```python
from build123d import *

# Parameters (mm, degrees)
EXTRUDE_1_DEPTH     = 332
SKETCH_2_R          = 3.25
CUT_EXTRUDE_1_DEPTH = 5
SKETCH_3_R          = 5
CUT_EXTRUDE_2_DEPTH = 5
SKETCH_4_W          = 26.179083289
SKETCH_4_H          = 3.25731829
CUT_EXTRUDE_3_DEPTH = 10
SKETCH_5_R          = 1.75
CUT_EXTRUDE_4_DEPTH = 2.5
CHAMFER_1_SIZE      = 1.5
SKETCH_6_R          = 2.1
SKETCH_6_R_2        = 6
CUT_EXTRUDE_5_DEPTH = 10
SKETCH_8_R          = 2.1
SKETCH_8_R_2        = 1.1
CUT_EXTRUDE_6_DEPTH = 10
SKETCH_9_R          = 1.6
CUT_EXTRUDE_7_DEPTH = 10
CHAMFER_2_SIZE      = 1.5
SKETCH_10_R         = 2.1
CUT_EXTRUDE_8_DEPTH = 10


with BuildPart() as part:
    # Эскиз1 → Вытянуть1 (new body)
    with BuildSketch(Plane.XY):
        with BuildLine():
            Line((-1, -68), (-1, 104))
            ThreePointArc((-1, 104), (0.171572875, 106.828427125), (3, 108))
            Line((3, 108), (24, 108))
            Line((24, 108), (24, 106))
            Line((24, 106), (3, 106))
            ThreePointArc((3, 106), (1.585786438, 105.414213562), (1, 104))
            Line((1, 104), (1, -68))
            ThreePointArc((1, -68), (-0.171572875, -70.828427125), (-3, -72))
            Line((-3, -72), (-44, -72))
            Line((-44, -72), (-44, -70))
            Line((-44, -70), (-3, -70))
            ThreePointArc((-3, -70), (-1.585786438, -69.414213562), (-1, -68))
        make_face()
    extrude(amount=EXTRUDE_1_DEPTH)

    # Эскиз2 → Вырез-Вытянуть1 (cut)
    with BuildSketch(Plane.ZY.offset(1)):
        with Locations((31, -38)):
            Circle(SKETCH_2_R)
        with Locations((121, -38)):
            Circle(SKETCH_2_R)
        with Locations((211, -38)):
            Circle(SKETCH_2_R)
        with Locations((301, -38)):
            Circle(SKETCH_2_R)
    extrude(amount=-CUT_EXTRUDE_1_DEPTH, mode=Mode.SUBTRACT)

    # Эскиз3 → Вырез-Вытянуть2 (cut)
    with BuildSketch(Plane(origin=(0, -70, 0), x_dir=(1, 0, 0), z_dir=(0, 1, 0))):
        with Locations(Location((-24, -18.5, 0), (0, 0, 270))):
            Circle(SKETCH_3_R)
        with Locations(Location((-24, -313.5, 0), (0, 0, 270))):
            Circle(SKETCH_3_R)
    extrude(amount=-CUT_EXTRUDE_2_DEPTH, mode=Mode.SUBTRACT)

    # Эскиз4 → Вырез-Вытянуть3 (cut)
    with BuildSketch(Plane(origin=(0, 108, 0), x_dir=(1, 0, 0), z_dir=(0, 1, 0))):
        with Locations((16.089541645, 0.628659145)):
            Rectangle(SKETCH_4_W, SKETCH_4_H)
        with Locations((16.089541645, -332.628659145)):
            Rectangle(SKETCH_4_W, SKETCH_4_H)
    extrude(amount=-CUT_EXTRUDE_3_DEPTH, mode=Mode.SUBTRACT)

    # Эскиз5 → Вырез-Вытянуть4 (cut)
    with BuildSketch(Plane.ZY.offset(1)):
        with Locations(Location((5.7, 95, 0), (0, 0, 270))):
            Circle(SKETCH_5_R)
        with Locations(Location((326.3, 95, 0), (0, 0, 270))):
            Circle(SKETCH_5_R)
    extrude(amount=-CUT_EXTRUDE_4_DEPTH, mode=Mode.SUBTRACT)

    # Фаска1
    chamfer_1_edges = [part.edges().sort_by_distance(p)[0] for p in [
        (-1, 96.75, 326.3),
        (-1, 96.75, 5.7),
    ]]
    chamfer(chamfer_1_edges, length=CHAMFER_1_SIZE)

    # Эскиз6 → Вырез-Вытянуть5 (cut)
    with BuildSketch(Plane.ZY.offset(1)):
        with Locations(Location((47, 91, 0), (0, 0, 270))):
            Circle(SKETCH_6_R)
        with Locations(Location((47, 41, 0), (0, 0, 270))):
            Circle(SKETCH_6_R)
        with Locations(Location((47, 31, 0), (0, 0, 270))):
            Circle(SKETCH_6_R)
        with Locations(Location((47, -19, 0), (0, 0, 270))):
            Circle(SKETCH_6_R)
        with Locations(Location((45, -1.5, 0), (0, 0, 270))):
            Circle(SKETCH_6_R_2)
        with Locations(Location((45, 58.5, 0), (0, 0, 270))):
            Circle(SKETCH_6_R_2)
        with Locations(Location((45, 13.5, 0), (0, 0, 270))):
            Circle(SKETCH_6_R_2)
        with Locations(Location((45, 73.5, 0), (0, 0, 270))):
            Circle(SKETCH_6_R_2)
    extrude(amount=-CUT_EXTRUDE_5_DEPTH, mode=Mode.SUBTRACT)

    # Эскиз8 → Вырез-Вытянуть6 (cut)
    with BuildSketch(Plane.ZY.offset(1)):
        with Locations(Location((267, -20, 0), (0, 0, 270))):
            Circle(SKETCH_8_R)
        with Locations(Location((287, 15, 0), (0, 0, 270))):
            Circle(SKETCH_8_R_2)
        with Locations(Location((247, 15, 0), (0, 0, 270))):
            Circle(SKETCH_8_R_2)
        with BuildLine():
            Line((255.5, 5), (278.5, 5))
            ThreePointArc((278.5, 5), (280.267766953, 5.732233047), (281, 7.5))
            Line((281, 7.5), (281, 22.5))
            ThreePointArc((281, 22.5), (280.267766953, 24.267766953), (278.5, 25))
            Line((278.5, 25), (255.5, 25))
            ThreePointArc((255.5, 25), (253.732233047, 24.267766953), (253, 22.5))
            Line((253, 22.5), (253, 7.5))
            ThreePointArc((253, 7.5), (253.732233047, 5.732233047), (255.5, 5))
        make_face()
    extrude(amount=-CUT_EXTRUDE_6_DEPTH, mode=Mode.SUBTRACT)

    # Эскиз9 → Вырез-Вытянуть7 (cut)
    with BuildSketch(Plane(origin=(0, 108, 0), x_dir=(1, 0, 0), z_dir=(0, 1, 0))):
        with Locations(Location((14, -266, 0), (0, 0, 270))):
            Circle(SKETCH_9_R)
        with Locations(Location((14, -292, 0), (0, 0, 270))):
            Circle(SKETCH_9_R)
    extrude(amount=-CUT_EXTRUDE_7_DEPTH, mode=Mode.SUBTRACT)

    # Фаска2
    chamfer_2_edges = [part.edges().sort_by_distance(p)[0] for p in [
        (14, 108, 264.4),
        (14, 108, 290.4),
    ]]
    chamfer(chamfer_2_edges, length=CHAMFER_2_SIZE)

    # Эскиз10 → Вырез-Вытянуть8 (cut)
    with BuildSketch(Plane(origin=(0, 108, 0), x_dir=(1, 0, 0), z_dir=(0, 1, 0))):
        with Locations(Location((13, -15, 0), (0, 0, 270))):
            Circle(SKETCH_10_R)
        with Locations(Location((13, -166, 0), (0, 0, 270))):
            Circle(SKETCH_10_R)
        with Locations(Location((13, -317, 0), (0, 0, 270))):
            Circle(SKETCH_10_R)
    extrude(amount=-CUT_EXTRUDE_8_DEPTH, mode=Mode.SUBTRACT)


solid = part.part
```
Can you work these out from the model? Positions are in its coordinate system, mm. A direction names the side the tool comes from. Coordinates: 2 decimals unless noted, no trailing zeros. Order: outer loops, then holes, each group sorted by start corner. A loop starts at its lowest first (then second) coordinate and runs counter-clockwise, first axis right, second up. Notation, with made-up numbers: (59, 60) -> (74, 60) arc R21 ccw to (74, 99) -> close; hole circle Ø10 at (87, 45). An arc over 180 degrees is marked (long way). Write each question's results on one line, items separated by ' | '.
Item 1: If I drill on line 1 along Z through (x, y) = (0.8, 95); line 2 along Z through (x, y) = (0, 41); line 3 along Z through (x, y) = (0, 95), over which ranges is the centre line in solid material (lowest first)?
Results are:
line 1: 0 to 3.95, 7.45 to 324.55, 328.05 to 332 | line 2: 0 to 44.9, 49.1 to 332 | line 3: 0 to 3.45, 7.95 to 324.05, 328.55 to 332
Item 2: I want a section at C-C, the plane z = 31. Write out the boundary of the cut face in (x, y), then the cut area to 3 significant figures.
Results are:
outline: (-44, -72) -> (-3, -72) arc R4 ccw to (1, -68) -> (1, -41.25) -> (-1, -41.25) -> (-1, -68) arc R2 cw to (-3, -70) -> (-44, -70) -> close; (-1, -34.75) -> (1, -34.75) -> (1, 104) arc R2 cw to (3, 106) -> (24, 106) -> (24, 108) -> (3, 108) arc R4 ccw to (-1, 104) -> close | area: 474 mm²
Item 3: If we mould it in two halves opening along Y, with no side actions, what happens to faces 3 (the face through (-0.014, -39.245, 214.002)), 4 (the face through (-23, -72, 164)), 5 (the face through (-24, -70, 164))? For each: +Y half, -Y half, draft (parallel to the pull), parting line (faces both ways), or undercut.
Results are:
face 3: undercut | face 4: -Y half | face 5: +Y half
Item 4: I want a section at A-A, the plane y = 58.5. Write out the boundary of the cut face in (x, z), then the cut area to 3 significant figures.
Results are:
outline: (-1, 0) -> (1, 0) -> (1, 39) -> (-1, 39) -> close; (-1, 51) -> (1, 51) -> (1, 332) -> (-1, 332) -> close | area: 640 mm²
Item 5: I want a section at D-D, the plane z = 143.5. Write out the boundary of the cut face in (x, y), then the cut area to 3 significant figures.
Results are:
outline: (-44, -72) -> (-3, -72) arc R4 ccw to (1, -68) -> (1, 104) arc R2 cw to (3, 106) -> (24, 106) -> (24, 108) -> (3, 108) arc R4 ccw to (-1, 104) -> (-1, -68) arc R2 cw to (-3, -70) -> (-44, -70) -> close | area: 487 mm²
Item 6: I want a section at B-B, the plane x = -24. Write out the boundary of the cut face in (y, z), then the cut area to 3 significant figures.
Results are:
outline: (-72, 0) -> (-70, 0) -> (-70, 13.5) -> (-72, 13.5) -> close; (-72, 23.5) -> (-70, 23.5) -> (-70, 308.5) -> (-72, 308.5) -> close; (-72, 318.5) -> (-70, 318.5) -> (-70, 332) -> (-72, 332) -> close | area: 624 mm²
Item 7: Which directions (+Z, -Z, +X, -X, +Y, -Y) give clear straight access to the entire face, cutting with the end or side of a thin tool? Please do faces 1 (the face through (1, 19, 164)), 2 (the face through (-0.014, -39.978, 298.421)).
Results are:
face 1: +Z, -Z, +X, -Y | face 2: +X, -X
Item 8: I'm going to push flat-ended pins straight in: pin 1 Ø3 at (x, z) = (-2, 265.5) entering from +Y; pin 2 Ø4 at (y, z) = (59.5, 240.5) entering from -X; pin 3 Ø3.5 at (x, z) = (14, 266) entering from -Y. Where does each tip first touch, or does it pass through?
Results are:
pin 1: y = 105.94 | pin 2: x = -1 | pin 3: y = 106
